Geometry check sheet. Reference: the model listing, model coordinates, mm. Face numbers are marked on the shaded views. A direction names the side the tool comes from. Round coordinates to 2 decimals unless told otherwise and drop trailing zeros. Order: outer loops, then holes, each group sorted by start corner. A loop starts at its lowest first (then second) coordinate and runs counter-clockwise, first axis right, second up.
(1) Gauge pin test, flat ends, axial feed: P1, Ø14.5, axis at x = -6.5, z = -20, coming from the +Y side; P2, Ø6, axis at y = 31.5, z = 19.5, coming from the +X side; P3, Ø13, axis at x = -21.5, z = 4.5, coming from the +Y side; P4, Ø20, axis at x = 11, z = -4.5, coming from the -Y side. Record the tip position at first contact, or that the pin passes through.
(2) Cross-section at A-A on y = 34.5. Enter the section's corners in (x, z), and give its area (3 significant figures).
(3) Draft check along X on the marked faces 1, 2 and 3. Enter one of: pulls with the +X half, pulls with the -X half, needs draft (parallel to the pull), parting line crosses it, or undercut.
(4) Thickness scan on L1, parallel to X at y = 1.5, z = 0; L2, parallel to X at y = 34.05, z = 0; L3, parallel to X at y = 33.5, z = 5. Record the ranges inside material, lowest first.
(5) Set-up check for the marked faces 4, 5 and 6: record each of +Z, -Z, +X, -X, +Y, -Y from which the full face is reachable in a straight line by a thin tool's end or side.
(6) Cross-section at B-B on y = 20. Enter the section's corners in (x, z), and give its area (3 significant figures).
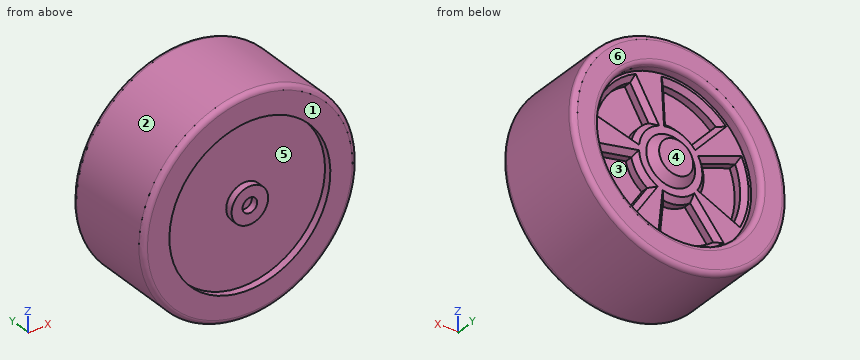
from build123d import *

# Parameters (mm, degrees)
SKETCH_1_R          = 44
EXTRUDE_1_DEPTH     = 38
SKETCH_3_R          = 33
CUT_EXTRUDE_1_DEPTH = 5
CUT_EXTRUDE_2_DEPTH = 5
SKETCH_5_R          = 10
EXTRUDE_2_DEPTH     = 3
CHAMFER_1_SIZE      = 3
CHAMFER_2_SIZE      = 2
FILLET_1_R          = 2
CUT_EXTRUDE_START   = -2.92
SKETCH_6_R          = 33
SKETCH_6_R_2        = 7.5
SKETCH_6_R_3        = 3
CUT_EXTRUDE_3_DEPTH = 2.92


with BuildPart() as part:
    # 草图1 → 凸台-拉伸1 (new body)
    with BuildSketch(Plane(origin=(0, 0, 0), x_dir=(1, 0, 0), z_dir=(0, 1, 0))):
        with Locations(Location((0, 0, 0), (0, 0, 270))):
            Circle(SKETCH_1_R)
    extrude(amount=EXTRUDE_1_DEPTH)

    # 草图3 → 切除-拉伸1 (cut)
    with BuildSketch(Plane(origin=(0, 38, 0), x_dir=(1, 0, 0), z_dir=(0, 1, 0))):
        with Locations(Location((0, 0, 0), (0, 0, 270))):
            Circle(SKETCH_3_R)
    extrude(amount=-CUT_EXTRUDE_1_DEPTH, mode=Mode.SUBTRACT)

    # 草图4 → 切除-拉伸2 (cut)
    with BuildSketch(Plane(origin=(0, 33, 0), x_dir=(1, 0, 0), z_dir=(0, 1, 0))):
        with BuildLine():
            Line((-18.971630185, 23.239562132), (-9.485815093, 11.619781066))
            ThreePointArc((-9.485815093, 11.619781066), (-4.317052712, 14.365342178), (1.508941811, 14.923910165))
            Line((1.508941811, 14.923910165), (3.017883621, 29.84782033))
            ThreePointArc((3.017883621, 29.84782033), (-8.634105423, 28.730684356), (-18.971630185, 23.239562132))
        make_face()
        with BuildLine():
            Line((29.319541348, 6.353305844), (14.659770674, 3.176652922))
            ThreePointArc((14.659770674, 3.176652922), (12.328209633, 8.544895976), (8.119790432, 12.612256077))
            Line((8.119790432, 12.612256077), (16.239580864, 25.224512153))
            ThreePointArc((16.239580864, 25.224512153), (24.656419267, 17.089791951), (29.319541348, 6.353305844))
        make_face()
        with BuildLine():
            Line((15.102589466, -25.921261378), (7.551294733, -12.960630689))
            ThreePointArc((7.551294733, -12.960630689), (11.936305286, -9.084306035), (14.504121561, -3.824978136))
            Line((14.504121561, -3.824978136), (29.008243122, -7.649956272))
            ThreePointArc((29.008243122, -7.649956272), (23.872610571, -18.168612069), (15.102589466, -25.921261378))
        make_face()
        with BuildLine():
            Line((-19.98562774, -22.373526406), (-9.99281387, -11.186763203))
            ThreePointArc((-9.99281387, -11.186763203), (-4.951167267, -14.159305869), (0.84424967, -14.976222571))
            Line((0.84424967, -14.976222571), (1.68849934, -29.952445142))
            ThreePointArc((1.68849934, -29.952445142), (-9.902334534, -28.318611738), (-19.98562774, -22.373526406))
        make_face()
        with BuildLine():
            Line((-27.454386696, 12.09366161), (-13.727193348, 6.046830805))
            ThreePointArc((-13.727193348, 6.046830805), (-14.996294941, 0.33337375), (-13.98234657, -5.430836436))
            Line((-13.98234657, -5.430836436), (-27.96469314, -10.861672872))
            ThreePointArc((-27.96469314, -10.861672872), (-29.992589881, 0.666747501), (-27.454386696, 12.09366161))
        make_face()
    extrude(amount=-CUT_EXTRUDE_2_DEPTH, mode=Mode.SUBTRACT)

    # 草图5 → 凸台-拉伸2 (add)
    with BuildSketch(Plane(origin=(0, 33, 0), x_dir=(1, 0, 0), z_dir=(0, 1, 0))):
        with Locations(Location((0, 0, 0), (0, 0, 270))):
            Circle(SKETCH_5_R)
    extrude(amount=EXTRUDE_2_DEPTH)

    # 倒角1
    chamfer_1_edges = [part.edges().sort_by_distance(p)[0] for p in [
        (0, 36, -10),
    ]]
    chamfer(chamfer_1_edges, length=CHAMFER_1_SIZE - 0.0001)  # a hair under: the kernel refuses the full size

    # 倒角2
    chamfer_2_edges = [part.edges().sort_by_distance(p)[0] for p in [
        (-14.996294941, 33, -0.33337375),
        (-20.590790022, 33, -9.070246208),
        (-29.992589881, 33, -0.666747501),
        (-20.973519855, 33, 8.146254654),
        (-4.951167267, 33, 14.159305869),
        (-14.989220805, 33, 16.780144805),
        (-9.902334534, 33, 28.318611738),
        (1.266374505, 33, 22.464333856),
        (11.936305286, 33, 9.084306035),
        (11.3269421, 33, 19.440946033),
        (23.872610571, 33, 18.168612069),
        (21.756182342, 33, 5.737467204),
        (12.328209633, 33, -8.544895976),
        (21.989656011, 33, -4.764979383),
        (24.656419267, 33, -17.089791951),
        (12.179685648, 33, -18.918384115),
        (-4.317052712, 33, -14.365342178),
        (2.263412716, 33, -22.385865247),
        (-8.634105423, 33, -28.730684356),
        (-14.228722639, 33, -17.429671599),
    ]]
    chamfer(chamfer_2_edges, length=CHAMFER_2_SIZE)

    # 圆角1
    fillet_1_edges = [part.edges().sort_by_distance(p)[0] for p in [
        (0, 0, -44),
        (0, 38, -44),
        (0, 38, -33),
    ]]
    fillet(fillet_1_edges, radius=FILLET_1_R)

    # 草图6 → 切除-拉伸3 (cut)
    # profile 1 of 2: a face of its own
    with BuildSketch(Plane.XZ.offset(CUT_EXTRUDE_START)):
        with Locations(Location((0, 0, 0), (0, 0, 90))):
            Circle(SKETCH_6_R)
        with Locations(Location((0, 0, 0), (0, 0, 270))):
            Circle(SKETCH_6_R_2, mode=Mode.SUBTRACT)
    # profile 2 of 2: a face of its own
    with BuildSketch(Plane.XZ.offset(CUT_EXTRUDE_START)):
        with Locations(Location((0, 0, 0), (0, 0, 270))):
            Circle(SKETCH_6_R_3)
    extrude(amount=CUT_EXTRUDE_3_DEPTH, mode=Mode.SUBTRACT)


solid = part.part
Found:
1. P1: stops at y = 32.22
1. P2: stops at x = 40.79
1. P3: stops at y = 33
1. P4: stops at y = 0
2. outline: circle Ø88 at (0, 0); circle Ø17 at (0, 0); hole circle Ø66 at (0, 0)
2. area: 2,890 mm2
3. face 1: needs draft
3. face 2: parting line crosses it
3. face 3: undercut
4. L1: x = -43.94 to -33, -7.5 to -3, 3 to 7.5, 33 to 43.94
4. L2: x = -44 to -33, -8.95 to 8.95, 33 to 44
4. L3: x = -43.71 to -32.62, -8.08 to 8.08, 32.62 to 43.71
5. face 4: +Y
5. face 5: -Y
5. face 6: +Z, -Z, +X, -X, +Y
6. outline: circle Ø88 at (0, 0)
6. area: 6,080 mm2
